Design review of the part built by this model. Coordinates are the model's own, in mm. A direction names the side the tool comes from. Round coordinates to 2 decimals unless told otherwise and drop trailing zeros. Order: outer loops, then holes, each group sorted by start corner. A loop starts at its lowest first (then second) coordinate and runs counter-clockwise, first axis right, second up.
from build123d import *

# Parameters (mm, degrees)
F0_W          = 17
F0_H          = 13
F0_W_2        = 12.7
F0_H_2        = 7
F0_R          = 1.1
F1_DEPTH      = 8
F2_W          = 15
F2_H          = 6
F3_DEPTH      = 4.501
F3_DEPTH_BACK = 3.5
F4_R          = 2.2
F5_DEPTH      = 9.301
F5_DEPTH_BACK = 7.701


with BuildPart() as f1:
    # F0 (on Top) → F1 (new body)
    with BuildSketch(Plane.XY):
        with Locations((-0.8, 2)):
            Rectangle(F0_W, F0_H)
        Rectangle(F0_W_2, F0_H_2, mode=Mode.SUBTRACT)
        Rectangle(F0_W_2, F0_H_2)
        with Locations((-3, -2.3)):
            Circle(F0_R, mode=Mode.SUBTRACT)
        with Locations((3, -2.3)):
            Circle(F0_R, mode=Mode.SUBTRACT)
    extrude(amount=F1_DEPTH)

    # F2 (on Front) → F3 (cut, two sides)
    with BuildSketch(Plane.XZ) as f3_sk:
        with Locations((-0.8, 3.7450972334)):
            Rectangle(F2_W, F2_H)
    extrude(amount=F3_DEPTH, mode=Mode.SUBTRACT)
    extrude(f3_sk.sketch, amount=-F3_DEPTH_BACK, mode=Mode.SUBTRACT)

    # F4 (on Right) → F5 (cut, two sides)
    with BuildSketch(Plane.YZ) as f5_sk:
        with Locations((3.5, 4)):
            Circle(F4_R)
    extrude(amount=-F5_DEPTH, mode=Mode.SUBTRACT)
    extrude(f5_sk.sketch, amount=F5_DEPTH_BACK, mode=Mode.SUBTRACT)


solid = f1.part
1) Take a section at D-D on y = 0.75. Give the boundary of the cut face in (x, z), plus the area to 3 significant figures.
Results:
outline: (-9.3, 0) - (7.7, 0) - (7.7, 8) - (-9.3, 8) - close; hole (-8.3, 0.75) - (6.7, 0.75) - (6.7, 6.75) - (-8.3, 6.75) - close
area: 46.0 mm2
2) The part is to be moulded in two halves that separate along Y. For faces 3 (the face through (-1.984, -2.721, 0.367)), 4 (the face through (-1, 8.5, 4)), 5 (the face through (0, -4.5, 7)), 6 (the face through (6.7, -1, 4)), say which applies: released by +Y, released by -Y, zero draft, split by the parting line, or undercut.
Results:
face 3: undercut
face 4: released by +Y
face 5: released by -Y
face 6: zero draft
3) Take a section at B-B on z = 4. Give the boundary of the cut face in (x, y), plus the area to 3 significant figures.
Results:
outline: (-9.3, -4.5) - (-8.3, -4.5) - (-8.3, 1.3) - (-9.3, 1.3) - close; (-9.3, 5.7) - (7.7, 5.7) - (7.7, 8.5) - (-9.3, 8.5) - close; (6.7, -4.5) - (7.7, -4.5) - (7.7, 1.3) - (6.7, 1.3) - close
area: 59.2 mm2
4) To check wall thickness, follow line 1 along X through (y, z) = (-2.3, 0.6); line 2 along Z through (x, y) = (-6, -1.25); line 3 along X through (y, z) = (-3.25, 7). State the ranges of each line that lie inside material, in increasing order.
Results:
line 1: x = -9.3 to -4.1, -1.9 to 1.9, 4.1 to 7.7
line 2: z = 0 to 0.75, 6.75 to 8
line 3: x = -9.3 to -3.55, -2.45 to 2.45, 3.55 to 7.7
5) For faces 1 (the face through (-8.3, -1, 4)), 2 (the face through (7.7, 0, 4)), list the 3-axis set-ups (+Z, -Z, +X, -X, +Y, -Y) from which the entire face can be reached by the end or side of a thin tool; tool diameter is ignored.
Results:
face 1: -Y
face 2: +Z, -Z, +X, +Y, -Y
6) Take a section at A-A on y = -2.3. Give the boundary of the cut face in (x, z).
Results:
outline: (-9.3, 0) - (-4.1, 0) - (-4.1, 0.75) - (-8.3, 0.75) - (-8.3, 6.75) - (-4.1, 6.75) - (-4.1, 8) - (-9.3, 8) - close; (-1.9, 0) - (1.9, 0) - (1.9, 0.75) - (-1.9, 0.75) - close; (-1.9, 6.75) - (1.9, 6.75) - (1.9, 8) - (-1.9, 8) - close; (4.1, 0) - (7.7, 0) - (7.7, 8) - (4.1, 8) - (4.1, 6.75) - (6.7, 6.75) - (6.7, 0.75) - (4.1, 0.75) - close
7) Take a section at C-C on x = -3. Give the boundary of the cut face in (y, z), plus the area to 3 significant figures.
Results:
outline: (-4.5, 0) - (-3.4, 0) - (-3.4, 0.75) - (-4.5, 0.75) - close; (-4.5, 6.75) - (-3.4, 6.75) - (-3.4, 8) - (-4.5, 8) - close; (-1.2, 0) - (8.5, 0) - (8.5, 8) - (-1.2, 8) - (-1.2, 6.75) - (3.5, 6.75) - (3.5, 6.2) arc R2.2 cw to (3.5, 1.8) - (3.5, 0.75) - (-1.2, 0.75) - close
area: 44.0 mm2
